Read the model definition and answer for the solid it produces. Units are mm, in the model's axes. Coordinates: 2 decimals unless noted, no trailing zeros. Order: outer loops, then holes, each group sorted by start corner. A loop starts at its lowest first (then second) coordinate and runs counter-clockwise, first axis right, second up.
```python
from build123d import *

# Parameters (mm, degrees)
F0_W     = 88.9
F0_H     = 76.2
F1_DEPTH = 25.4
F2_R     = 19.05
F3_DEPTH = 25.4
F4_R     = 5.08


with BuildPart() as f1:
    # F0 (on Front) → F1 (new body)
    with BuildSketch(Plane.XZ):
        with Locations((-1.889126, -0.429428)):
            Rectangle(F0_W, F0_H)
    extrude(amount=F1_DEPTH)

    # F2 (on face) → F3 (cut)
    with BuildSketch(Plane.XZ.offset(25.4)):
        Circle(F2_R)
    extrude(amount=-F3_DEPTH, mode=Mode.SUBTRACT)

    # F4
    f4_edges = [f1.edges().sort_by_distance(p)[0] for p in [
        (-46.339126, -25.4, -0.429428),
        (-1.889126, -25.4, 37.670572),
        (42.560874, -25.4, -0.429428),
        (-1.889126, -25.4, -38.529428),
    ]]
    fillet(f4_edges, radius=F4_R)


solid = f1.part
```
1) A cutting plane is placed at B-B, the plane x = 14. Determine the outline of the cut face in (y, z).
A:
outline: (-25.4, -33.45) arc R5.08 ccw to (-20.32, -38.53) - (0, -38.53) - (0, -12.92) - (-25.4, -12.92) - close; (-25.4, 12.92) - (0, 12.92) - (0, 37.67) - (-20.32, 37.67) arc R5.08 ccw to (-25.4, 32.59) - close
2) A cutting plane is placed at A-A, the plane z = 0. Determine the outline of the cut face in (x, y).
A:
outline: (-46.34, -20.32) arc R5.08 ccw to (-41.26, -25.4) - (-19.05, -25.4) - (-19.05, 0) - (-46.34, 0) - close; (19.05, -25.4) - (37.48, -25.4) arc R5.08 ccw to (42.56, -20.32) - (42.56, 0) - (19.05, 0) - close
3) A cutting plane is placed at C-C, the plane y = -19. Determine the outline of the cut face in (x, z).
A:
outline: (-46.34, -38.53) - (42.56, -38.53) - (42.56, 37.67) - (-46.34, 37.67) - close; hole circle Ø38.1 at (0, 0)
4) Straight lines are drawn through the part: line 1 (Z direction, x = 0, y = -17.5); line 2 (X direction, y = -11, z = 5); line 3 (X direction, y = -20.75, z = 17). For each, find the intervals that lie inside material, in ascending order.
A:
line 1: z = -38.53 to -19.05, 19.05 to 37.67
line 2: x = -46.34 to -18.38, 18.38 to 42.56
line 3: x = -46.32 to -8.6, 8.6 to 42.54
5) A flat-ended cylindrical pin translates along its axis: pin 1 Ø12 at (x, z) = (2.5, 10.5) entering from -Y (3 decimals). Find the tip coordinate at first contact, or state that the pin passes through.
A:
pin 1: passes through
6) Determine the mould class of faces 1 (the cylindrical face through (-15.12, -12.88, -11.59)), 2 (the cylindrical face through (-1.267, -23.872, -37.081)), 3 (the flat face through (-46.339, -10, -1)) for opening direction X: pulls with the +X half, pulls with the -X half, needs draft (parallel to the pull), parting line crosses it, or undercut.
A:
face 1: undercut
face 2: needs draft
face 3: pulls with the -X half
